Check sheet for the modelled part. Datum: model origin and axes. Units: mm. A direction names the side the tool comes from. Give positions to 0.01 mm unless a question says otherwise; leave off trailing zeros. Write each loop counter-clockwise with the first axis right and the second up, starting at its lowest first coordinate (ties: lowest second). Pieces come first, ordered by that corner, then holes. Notation, with made-up numbers: (-32.5, -34) -> (4.5, -34) arc R16 cw to (4.5, -11) -> close; hole circle Ø2 at (-26, 1). An arc over 180 degrees is marked (long way). Answer as a JSON object with one key per item and string values.
from build123d import *

# Parameters (mm, degrees)
SKETCH2_W                       = 39
SKETCH2_H                       = 43
SKETCH2_R                       = 3.175
BOSS_EXTRUDE1_DEPTH             = 4
BOSS_EXTRUDE2_REACH             = 55.226
SKETCH3_R                       = 2.5
SKETCH3_R_2                     = 2.1
BOSS_EXTRUDE2_DIRECTION_2_REACH = 55.226
SKETCH5_W                       = 35
SKETCH5_H                       = 44.559224728
CUT_EXTRUDE2_DEPTH              = 64.576725301


with BuildPart() as part:
    # Sketch2 → Boss-Extrude1 (new body)
    with BuildSketch(Plane(origin=(0, 0, 0), x_dir=(1, 0, 0), z_dir=(0, 1, 0))):
        with Locations((19.5, 14.5)):
            Rectangle(SKETCH2_W, SKETCH2_H)
        with Locations(Location((19.5, 14.5, 0), (0, 0, 270))):
            Circle(SKETCH2_R, mode=Mode.SUBTRACT)
    extrude(amount=BOSS_EXTRUDE1_DEPTH)

    # Boss-Extrude2: up to this face of the body (flat: up to its plane)
    boss_extrude2_end = Plane(part.part.faces().sort_by_distance((19.5, 2, 7))[0])
    # Sketch3 → Boss-Extrude2 (add, up to the picked face)
    with BuildSketch(Plane.XY, mode=Mode.PRIVATE) as boss_extrude2_sk1:
        with BuildLine():
            Line((39, 4), (28.158657967, 31.815738403))
            ThreePointArc((28.158657967, 31.815738403), (26.321463094, 34.127874272), (23.5, 35))
            Line((23.5, 35), (15.5, 35))
            ThreePointArc((15.5, 35), (12.678536906, 34.127874272), (10.841342033, 31.815738403))
            Line((10.841342033, 31.815738403), (0, 4))
            Line((0, 4), (39, 4))
        make_face()
        with Locations(Location((15.5, 30, 0), (0, 0, 180))):
            Circle(SKETCH3_R, mode=Mode.SUBTRACT)
        with Locations(Location((23.5, 30, 0), (0, 0, 180))):
            Circle(SKETCH3_R, mode=Mode.SUBTRACT)
        with Locations(Location((23.5, 22, 0), (0, 0, 180))):
            Circle(SKETCH3_R, mode=Mode.SUBTRACT)
        with Locations(Location((15.5, 22, 0), (0, 0, 180))):
            Circle(SKETCH3_R, mode=Mode.SUBTRACT)
        with Locations(Location((19.5, 26, 0), (0, 0, 180))):
            Circle(SKETCH3_R_2, mode=Mode.SUBTRACT)
    boss_extrude2_tool1 = split(extrude(boss_extrude2_sk1.sketch, amount=BOSS_EXTRUDE2_REACH, mode=Mode.PRIVATE), bisect_by=boss_extrude2_end, keep=Keep.BOTH, mode=Mode.PRIVATE)
    add(boss_extrude2_tool1.solids().sort_by(Axis((19.5, 15.979018, 0), (0, 0, 1)))[0])

    # Boss-Extrude2 direction 2: up to this face of the body (flat: up to its plane)
    boss_extrude2_direction_2_end = Plane(part.part.faces().sort_by_distance((19.5, 2, -36))[0])
    # Sketch3 → Boss-Extrude2 direction 2 (add, up to the picked face)
    with BuildSketch(Plane.XY, mode=Mode.PRIVATE) as boss_extrude2_direction_2_sk1:
        with BuildLine():
            Line((39, 4), (28.158657967, 31.815738403))
            ThreePointArc((28.158657967, 31.815738403), (26.321463094, 34.127874272), (23.5, 35))
            Line((23.5, 35), (15.5, 35))
            ThreePointArc((15.5, 35), (12.678536906, 34.127874272), (10.841342033, 31.815738403))
            Line((10.841342033, 31.815738403), (0, 4))
            Line((0, 4), (39, 4))
        make_face()
        with Locations(Location((15.5, 30, 0), (0, 0, 180))):
            Circle(SKETCH3_R, mode=Mode.SUBTRACT)
        with Locations(Location((23.5, 30, 0), (0, 0, 180))):
            Circle(SKETCH3_R, mode=Mode.SUBTRACT)
        with Locations(Location((23.5, 22, 0), (0, 0, 180))):
            Circle(SKETCH3_R, mode=Mode.SUBTRACT)
        with Locations(Location((15.5, 22, 0), (0, 0, 180))):
            Circle(SKETCH3_R, mode=Mode.SUBTRACT)
        with Locations(Location((19.5, 26, 0), (0, 0, 180))):
            Circle(SKETCH3_R_2, mode=Mode.SUBTRACT)
    boss_extrude2_direction_2_tool1 = split(extrude(boss_extrude2_direction_2_sk1.sketch, amount=-BOSS_EXTRUDE2_DIRECTION_2_REACH, mode=Mode.PRIVATE), bisect_by=boss_extrude2_direction_2_end, keep=Keep.BOTH, mode=Mode.PRIVATE)
    add(boss_extrude2_direction_2_tool1.solids().sort_by(Axis((19.5, 15.979018, 0), (0, 0, -1)))[0])

    # Sketch5 → Cut-Extrude2 (cut, through all)
    with BuildSketch(Plane(origin=(0, 0, 0), x_dir=(0, 0, -1), z_dir=(1, 0, 0))):
        with Locations((14.5, 26.279612364)):
            Rectangle(SKETCH5_W, SKETCH5_H)
    extrude(amount=CUT_EXTRUDE2_DEPTH, mode=Mode.SUBTRACT)


solid = part.part
1. Sectioned sample at B-B, the plane x = 19.5. Enter the section's corners in (y, z) (3 decimals).
Determined:
{"outline": "(0, -36) -> (23.9, -36) -> (23.9, -32) -> (4, -32) -> (4, -17.675) -> (0, -17.675) -> close; (0, -11.325) -> (4, -11.325) -> (4, 3) -> (23.9, 3) -> (23.9, 7) -> (0, 7) -> close; (28.1, -36) -> (35, -36) -> (35, -32) -> (28.1, -32) -> close; (28.1, 3) -> (35, 3) -> (35, 7) -> (28.1, 7) -> close"}
2. Sectioned sample at C-C, the plane y = 22. Enter the section's corners in (x, z), plus the area to 3 significant figures.
Determined:
{"outline": "(7.02, -36) -> (13, -36) -> (13, -32) -> (7.02, -32) -> close; (7.02, 3) -> (13, 3) -> (13, 7) -> (7.02, 7) -> close; (18, -36) -> (21, -36) -> (21, -32) -> (18, -32) -> close; (18, 3) -> (21, 3) -> (21, 7) -> (18, 7) -> close; (26, -36) -> (31.98, -36) -> (31.98, -32) -> (26, -32) -> close; (26, 3) -> (31.98, 3) -> (31.98, 7) -> (26, 7) -> close", "area": "120 mm^2"}
3. Sectioned sample at D-D, the plane y = 11.5. Enter the section's corners in (x, z), plus the area to 3 significant figures.
Determined:
{"outline": "(2.92, -36) -> (36.08, -36) -> (36.08, -32) -> (2.92, -32) -> close; (2.92, 3) -> (36.08, 3) -> (36.08, 7) -> (2.92, 7) -> close", "area": "265 mm^2"}
4. Sectioned sample at A-A, the plane z = -14.5. Enter the section's corners in (x, y) (3 decimals), plus the area to 3 significant figures.
Determined:
{"outline": "(0, 0) -> (16.325, 0) -> (16.325, 4) -> (0, 4) -> close; (22.675, 0) -> (39, 0) -> (39, 4) -> (22.675, 4) -> close", "area": "131 mm^2"}
5. Access from +Z, -Z, +X, -X, +Y, -Y to the whole of each face (thin tool, end or side, straight path). Record for faces 1 (the face through (19, 4, -10)), 2 (the face through (20.45, 1.97, -11.47)).
Determined:
{"face 1": "+X, -X, +Y", "face 2": "+Y, -Y"}
6. Scan lines: L1, parallel to Y at x = 23.5, z = -34; L2, parallel to Z at x = 19, y = 33; L3, parallel to X at y = 22, z = 4. Record each from-to range of solid material in increasing order. Write a range as [from, to].
Determined:
{"L1": "[0, 19.5], [24.5, 27.5], [32.5, 35]", "L2": "[-36, -32], [3, 7]", "L3": "[7.02, 13], [18, 21], [26, 31.98]"}
7. Mould release check, pull along Y, two halves, no side actions. Record for faces 3 (the face through (0, 2, -14)), 4 (the face through (5.497, 18.103, 5.028)), 5 (the face through (15.83, 27.52, 5.03)): released by +Y, released by -Y, zero draft, split by the parting line, or undercut.
Determined:
{"face 3": "zero draft", "face 4": "released by +Y", "face 5": "undercut"}
8. Go/stop test with a flat-tipped pin: P1, Ø1.5, axis at x = 21.5, z = -20.5, coming from the +Y side. Record where the tip stops, or that it passes through.
Determined:
{"P1": "y = 4"}
